Design review of the part built by this model. Coordinates are the model's own, in mm. Give positions to 0.01 mm unless a question says otherwise; leave off trailing zeros. Loops run counter-clockwise (first coordinate to the right, second up) from the corner with the lowest first, then second, coordinate; pieces in that order, holes last. Notation, with made-up numbers: (-30, 7.5) -> (4, 7.5) arc R7 ccw to (4, 11.5) -> close; hole circle Ø9 at (22.5, 63.5). An arc over 180 degrees is marked (long way). Use CSV: the item, a comma, the result in double quotes. Start each with the question number.
Item 1: Clearance check with flat-ended pins moving along their axes: pin 1 (4 mm diameter, centred on x = 2.5, z = 116, fed in from +Y); pin 2 (5.5 mm diameter, centred on x = 0, y = 0, fed in from +Z); pin 3 (5 mm diameter, centred on x = 0, z = 115, fed in from +Y). State where each tip first meets the part, or that it passes through.
Item 2: Wall thickness on line 1 along Z through (x, y) = (0, 5.5); line 2 along Z through (x, y) = (-0.5, -4); line 3 along X through (y, z) = (2.75, -115): over which ranges is each line inside the solid? List them lowest first. Write a range as from..to.
Item 3: We need section A-A (z = -115). State the section outline as (x, y) points.
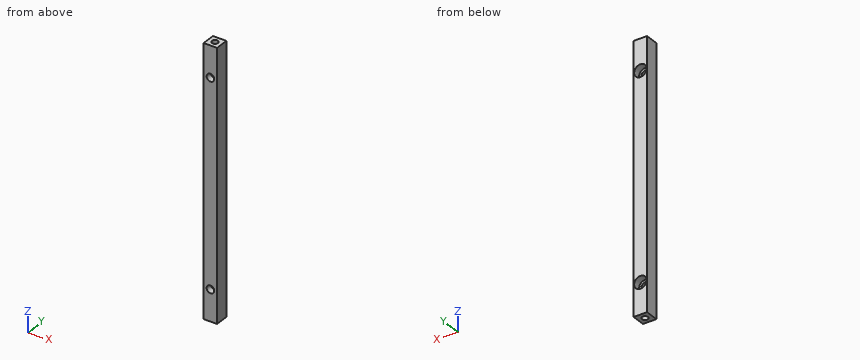
from build123d import *

# Parameters (mm, degrees)
IZIM1_W                     = 15
IZIM1_H                     = 15
Y_KSEKLIK_EKSTR_ZYON1_DEPTH = 150
DELIK1_D                    = 8.5
DELIK1_DEPTH                = 15
DELIK1_CBORE_D              = 14
DELIK1_CBORE_DEPTH          = 8


with BuildPart() as part:
    # Çizim1 → Yükseklik-Ekstrüzyon1 (new body, symmetric)
    with BuildSketch(Plane.XY):
        Rectangle(IZIM1_W, IZIM1_H)
    extrude(amount=Y_KSEKLIK_EKSTR_ZYON1_DEPTH, both=True)

    # Çizim3 → M8 Dişli Delik1 (revolve, cut)
    with BuildSketch(Plane(origin=(0, 0, 150), x_dir=(0, -1, 0), z_dir=(1, 0, 0))):
        Polygon((0, 0), (0, 24.292926105), (3.4, 22.25), (3.4, 0), align=None)
    m8_di_li_delik1 = revolve(axis=Axis((0, 0, 156.35), (0, 0, -1)), mode=Mode.SUBTRACT)

    # Aynalama1: M8 Dişli Delik1 across plane
    add(m8_di_li_delik1.mirror(Plane.XY), mode=Mode.SUBTRACT)

    # Delik1
    with Locations(Plane(origin=(0, 7.5, 0), x_dir=(1, 0, 0), z_dir=(0, 1, 0))):
        with Locations((0, 115)):
            delik1 = CounterBoreHole(DELIK1_D / 2, DELIK1_CBORE_D / 2, DELIK1_CBORE_DEPTH, depth=DELIK1_DEPTH)

    # Aynalama2: Delik1 across plane
    add(delik1.mirror(Plane.XY), mode=Mode.SUBTRACT)


solid = part.part
Results found:
1,pin 1,"y = -0.5"
1,pin 2,"z = 127.36"
1,pin 3,"through"
2,line 1,"-150..-122, -108..108, 122..150"
2,line 2,"-150..-119.22, -110.78..110.78, 119.22..150"
2,line 3,"-7.5..-7, 7..7.5"
3,outline,"(-7.5, -7.5) -> (-4.25, -7.5) -> (-4.25, -0.5) -> (-7, -0.5) -> (-7, 7.5) -> (-7.5, 7.5) -> close; (4.25, -7.5) -> (7.5, -7.5) -> (7.5, 7.5) -> (7, 7.5) -> (7, -0.5) -> (4.25, -0.5) -> close"
